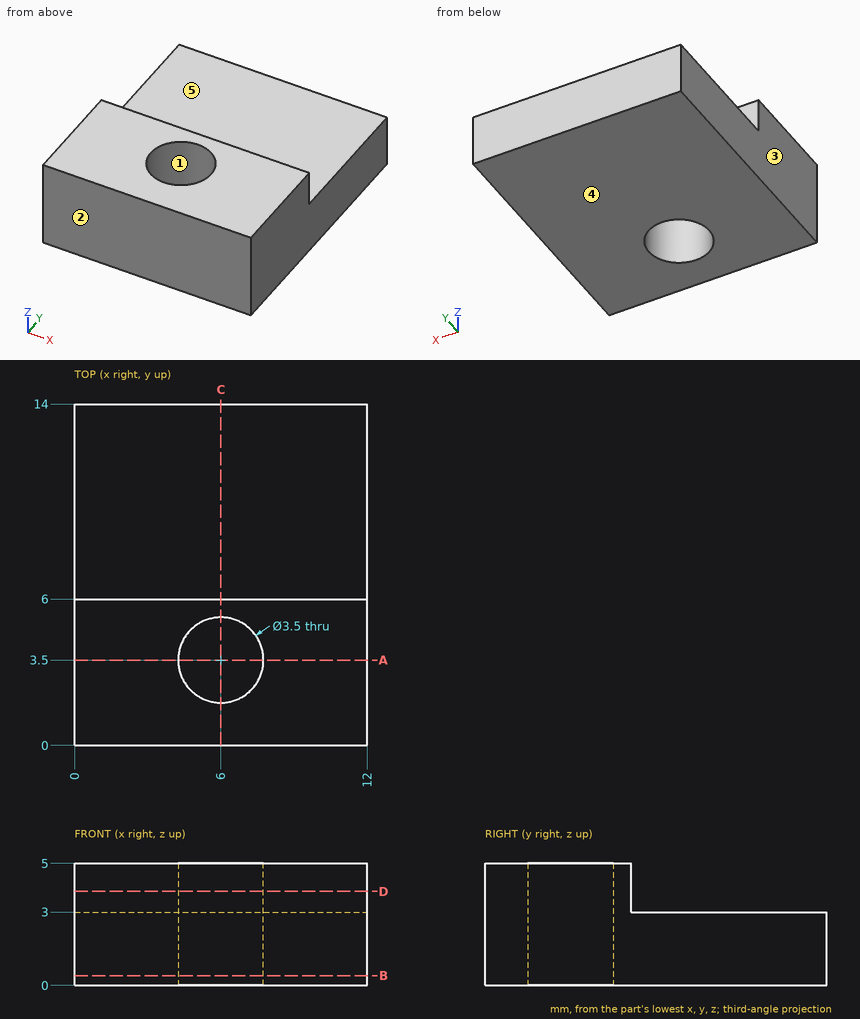
Could you check a few things on this drawing? It's one solid part, dimensions in mm from its lowest x, y, z. A direction names the side the tool comes from. Coordinates: 2 decimals unless noted, no trailing zeros. Order: outer loops, then holes, each group sorted by start corner. A loop starts at its lowest first (then second) coordinate and runs counter-clockwise, first axis right, second up.
1) Imagine slicing it at B-B on z = 0.4. List the corners of the cut face in (x, y) for me, and give its area (3 significant figures).
2) Imagine slicing it at A-A on y = 3.5. List the corners of the cut face in (x, z) for me, and give its area (3 significant figures).
3) Which directions (+Z, -Z, +X, -X, +Y, -Y) give clear straight access to the entire face, cutting with the end or side of a thin tool? Please do the marked faces 4 and 5.
4) Imagine slicing it at D-D on z = 3.85. List the corners of the cut face in (x, y) for me.
5) I need wall thicknesses on line 1 (Y direction, x = 6, z = 3.6); line 2 (Z direction, x = 9, y = 9); line 3 (Y direction, x = 6, z = 2.3). Which ranges of each line are inside material? Lowest first, please.
6) Imagine slicing it at C-C on x = 6. List the corners of the cut face in (y, z) for me.
7) Will these pins go through, and if not, where does the flat tip stop? pin 1 (5 mm diameter, centred on x = 3, y = 12, fed in from +Z); pin 2 (1.6 mm diameter, centred on x = 4, z = 4, fed in from +Y).
8) We'd pull the mould along X, two halves only. Please class the marked faces 1, 2 and 3: +X half, -X half, draft (parallel to the pull), parting line (faces both ways), or undercut.
Response values:
1. outline: (0, 0) - (12, 0) - (12, 14) - (0, 14) - close; hole circle Ø3.5 at (6, 3.5)
1. area: 158 mm2
2. outline: (0, 0) - (4.25, 0) - (4.25, 5) - (0, 5) - close; (7.75, 0) - (12, 0) - (12, 5) - (7.75, 5) - close
2. area: 42.5 mm2
3. face 4: -Z, +X, -X, +Y, -Y
3. face 5: +Z, +X, -X, +Y
4. outline: (0, 0) - (12, 0) - (12, 6) - (0, 6) - close; hole circle Ø3.5 at (6, 3.5)
5. line 1: y = 0 to 1.75, 5.25 to 6
5. line 2: z = 0 to 3
5. line 3: y = 0 to 1.75, 5.25 to 14
6. outline: (0, 0) - (1.75, 0) - (1.75, 5) - (0, 5) - close; (5.25, 0) - (14, 0) - (14, 3) - (6, 3) - (6, 5) - (5.25, 5) - close
7. pin 1: stops at z = 3
7. pin 2: stops at y = 6
8. face 1: undercut
8. face 2: draft
8. face 3: -X half
